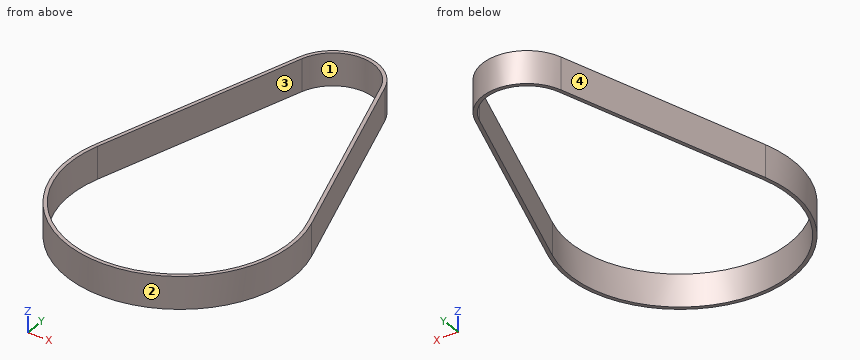
Autodesk Inventor part; units mm, degrees
ref_plane "YZ Plane" through (0, 0, 0) normal (1, 0, 0) x (0, 1, 0)
ref_plane "XZ Plane" through (0, 0, 0) normal (0, 1, 0) x (-1, 0, 0)
ref_plane "XY Plane" through (0, 0, 0) normal (0, 0, 1) x (1, 0, 0)
sketch "Sketch1" plane through (0, 0, 0) normal (0, 0, 1) x (1, 0, 0)
  arc A0 (0, 30.55) -> (-29.1137, 9.2571) centre (0, 0) ccw construction
  arc A1 (0, 51.5833) -> (10.9117, 66.5028) centre (0, 63.0333) ccw construction
  line L0 (10.9117, 66.5028) -> (29.1137, 9.2571)
  line L1 (-10.9117, 66.5028) -> (-29.1137, 9.2571)
  line L2 (0, 63.0333) -> (0, 0) construction
  arc A2 (-10.9117, 66.5028) -> (0, 51.5833) centre (0, 63.0333) ccw construction
  arc A3 (10.9117, 66.5028) -> (-10.9117, 66.5028) centre (0, 63.0333) ccw
  arc A4 (29.1137, 9.2571) -> (0, 30.55) centre (0, 0) ccw construction
  arc A5 (-29.1137, 9.2571) -> (29.1137, 9.2571) centre (0, 0) ccw
  arc A6 (-11.8647, 66.8058) -> (11.8647, 66.8058) centre (0, 63.0333) ccw construction
  arc A7 (30.0667, 9.5601) -> (-30.0667, 9.5601) centre (0, 0) ccw construction
  line L3 (-11.8647, 66.8058) -> (-30.0667, 9.5601)
  line L4 (11.8647, 66.8058) -> (30.0667, 9.5601)
  arc A8 (11.8647, 66.8058) -> (-11.8647, 66.8058) centre (0, 63.0333) ccw
  arc A9 (-30.0667, 9.5601) -> (30.0667, 9.5601) centre (0, 0) ccw
  dimension "d0" = 60.0698
  dimension "d1" = 22.9
  dimension "d2" = 61.1
  dimension "d3" = 24.9
  dimension "d4" = 63.1
extrude "Extrusion1" add sketch "Sketch1" along normal blind 9
ref_plane "Work Plane1" through (0, 0, 4.5) normal (0, 0, 1) x (1, 0, 0)
properties part number "Timming Belt - 165"
The listing builds one solid part. Answer for the finished solid, in the listing's coordinates (mm). Face numbers are marked on the shaded views. Round coordinates to 2 decimals unless told otherwise and drop trailing zeros. Write each loop counter-clockwise with the first axis right and the second up, starting at its lowest first coordinate (ties: lowest second). Pieces come first, ordered by that corner, then holes. Notation, with made-up numbers: (5.25, -22.75) -> (62.25, -22.75) arc R10 ccw to (62.25, -13.75) -> close; hole circle Ø10 at (21, -10.5). An arc over 180 degrees is marked (long way). Answer as a JSON object with one key per item and string values. Group by question number.
Q1. Straight lines are drawn through the part: line 1 along X through (y, z) = (0, 5.25); line 2 along X through (y, z) = (7, 5); line 3 along Y through (x, z) = (6.5, 6.5). For each, find the intervals that lie inside material, in ascending order.
Q2. Determine the mould class of the marked faces 1, 2, 3 and 4 for opening direction Y: pulls with the +Y half, pulls with the -Y half, needs draft (parallel to the pull), parting line crosses it, or undercut.
Q3. Section C-C (x = 0) is taken. Write down the section's boundary in (y, z), plus the area to 3 significant figures.
Q4. Section A-A (y = 0) is taken. Write down the section's boundary in (x, z).
Q5. Section B-B (z = 4) is taken. Write down the section's boundary in (x, y), plus the area to 3 significant figures.
Q6. This flat-tipped pin is pushed along its axis until it touches: pin 1 Ø5 at (y, z) = (44, 5) entering from -X. Where does it stop, or does it pass through?
Check values:
{
 "1": {"line 1": "-31.55 to -30.55, 30.55 to 31.55", "line 2": "-30.76 to -29.74, 29.74 to 30.76", "line 3": "-30.87 to -29.85, 72.46 to 73.65"},
 "2": {"face 1": "undercut", "face 2": "parting line crosses it", "face 3": "undercut", "face 4": "pulls with the +Y half"},
 "3": {"outline": "(-31.55, 0) -> (-30.55, 0) -> (-30.55, 9) -> (-31.55, 9) -> close; (74.48, 0) -> (75.48, 0) -> (75.48, 9) -> (74.48, 9) -> close", "area": "18.0 mm^2"},
 "4": {"outline": "(-31.55, 0) -> (-30.55, 0) -> (-30.55, 9) -> (-31.55, 9) -> close; (30.55, 0) -> (31.55, 0) -> (31.55, 9) -> (30.55, 9) -> close"},
 "5": {"outline": "(-30.07, 9.56) arc R31.55 ccw (long way) to (30.07, 9.56) -> (11.86, 66.81) arc R12.45 ccw to (-11.86, 66.81) -> close; hole (-29.11, 9.26) arc R30.55 ccw (long way) to (29.11, 9.26) -> (10.91, 66.5) arc R11.45 ccw to (-10.91, 66.5) -> close", "area": "267 mm^2"},
 "6": {"pin 1": "x = -19.91"}
}
